Model file for the job. Use its own axes, mm. A direction names the side the tool comes from. Give positions to 0.01 mm unless a question says otherwise; leave off trailing zeros. Loops run counter-clockwise (first coordinate to the right, second up) from the corner with the lowest first, then second, coordinate; pieces in that order, holes last. Notation, with made-up numbers: (13.25, 63.25) -> (42.25, 63.25) arc R30 ccw to (42.25, 96.25) -> close; hole circle Ø9 at (-7.5, 18.25). An arc over 180 degrees is marked (long way). Use CSV: the item, a comma, the result in double quotes. Start each with the question number.
(1) Drill centre lines: probe 1 along Z at (x, y) = (-5.5, 0.25); probe 2 along Y at (x, z) = (0, 8); probe 3 along X at (y, z) = (2, 7.25). Where is each one in solid material? Low to high.
(2) 3-axis set-ups, long thin cutter, end or side, ignore diameter. For faces 1 (the cylindrical face through (-0.45, 4.62, 1.82)), 2 (the cylindrical face through (-2.38, 3.82, 10.44)), 3 (the cylindrical face through (-6.466, 2.681, 3.204)), 4 (the cylindrical face through (0, -4.5, 10.4)): which of +Z, -Z, +X, -X, +Y, -Y reach the whole face in a straight line?
(3) Cut at A-A on x = 0. Write the cut outline in (y, z), then the cut area to 3 significant figures.
(4) Cut at C-C on y = -2.25. Write the cut outline in (x, z).
(5) Pull direction Z, two halves, no side cores. Call faces 5 (the flat face through (-3, 0, 16)), 6 (the cylindrical face through (-6.466, 2.681, 15.24)), 7 (the cylindrical face through (-0.841, 4.422, 10.444)): pulls with the +Z half, pulls with the -Z half, needs draft (parallel to the pull), parting line crosses it, or undercut.
(6) Flat gauge pins, fed straight in: pin 1 (7 mm diameter, centred on x = -1, y = 0, fed in from +Z); pin 2 (2 mm diameter, centred on x = -3, z = 14, fed in from +Y); pin 3 (6 mm diameter, centred on x = 3.5, z = 5.5, fed in from +Y); pin 4 (1.8 mm diameter, centred on x = 0, z = 3.25, fed in from +Y). Where does each tip first touch, or does it go through?
(7) Cut at B-B on y = 5.5. Write the cut outline in (x, z), then the cut area to 3 significant figures.
(8) Cut at D-D on x = -5.75. Write the cut outline in (y, z), then the cut area to 3 significant figures.
from build123d import *

# Parameters (mm, degrees)
ESQUISSE1_R                  = 7
BOSS_EXTRU_1_DEPTH           = 6.5
BOSS_EXTRU_2_DEPTH           = 8
ESQUISSE4_R                  = 7
BOSS_EXTRU_3_DEPTH           = 1.5
ESQUISSE5_R                  = 2.75
ENL_V_MAT_EXTRU_1_DEPTH      = 16
ENL_V_MAT_EXTRU_3_REACH      = 20.815
ENL_V_MAT_EXTRU_3_END_RADIUS = 7
ESQUISSE8_R                  = 1.5


with BuildPart() as part:
    # Esquisse1 → Boss.-Extru.1 (new body)
    with BuildSketch(Plane.XY):
        with Locations(Location((0, 0, 0), (0, 0, 180))):
            Circle(ESQUISSE1_R)
    extrude(amount=BOSS_EXTRU_1_DEPTH)

    # Esquisse3 → Boss.-Extru.2 (add)
    with BuildSketch(Plane.XY.offset(6.5)):
        with BuildLine():
            Line((0, 5.194220739), (0.3, 5.194220739))
            ThreePointArc((0.3, 5.194220739), (0.827122819, 4.424716273), (1.596627286, 4.951839093))
            Line((1.596627286, 4.951839093), (1.876368954, 4.843466593))
            Line((1.876368954, 4.843466593), (2.156110623, 4.735094093))
            ThreePointArc((2.156110623, 4.735094093), (2.369660938, 3.827133822), (3.277621209, 4.040684138))
            Line((3.277621209, 4.040684138), (3.499323884, 3.838575444))
            Line((3.499323884, 3.838575444), (3.721026559, 3.636466751))
            ThreePointArc((3.721026559, 3.636466751), (3.592163217, 2.712675742), (4.515954226, 2.583812399))
            Line((4.515954226, 2.583812399), (4.649675733, 2.315263412))
            Line((4.649675733, 2.315263412), (4.78339724, 2.046714425))
            ThreePointArc((4.78339724, 2.046714425), (4.329523948, 1.231855771), (5.144382602, 0.777982479))
            Line((5.144382602, 0.777982479), (5.172063109, 0.479262226))
            Line((5.172063109, 0.479262226), (5.199743617, 0.180541973))
            ThreePointArc((5.199743617, 0.180541973), (4.482158479, -0.415333148), (5.0780336, -1.132918286))
            Line((5.0780336, -1.132918286), (4.995934703, -1.421465979))
            Line((4.995934703, -1.421465979), (4.913835806, -1.710013672))
            ThreePointArc((4.913835806, -1.710013672), (4.029452671, -2.006429023), (4.325868023, -2.890812158))
            Line((4.325868023, -2.890812158), (4.145077632, -3.130217327))
            Line((4.145077632, -3.130217327), (3.964287241, -3.369622495))
            ThreePointArc((3.964287241, -3.369622495), (3.032546952, -3.326545541), (2.989469999, -4.258285831))
            Line((2.989469999, -4.258285831), (2.734404858, -4.416215479))
            Line((2.734404858, -4.416215479), (2.479339718, -4.574145128))
            ThreePointArc((2.479339718, -4.574145128), (1.626078963, -4.197393651), (1.249327486, -5.050654405))
            Line((1.249327486, -5.050654405), (0.954435556, -5.105779261))
            Line((0.954435556, -5.105779261), (0.659543626, -5.160904116))
            ThreePointArc((0.659543626, -5.160904116), (0, -4.50136049), (-0.659543626, -5.160904116))
            Line((-0.659543626, -5.160904116), (-0.954435556, -5.105779261))
            Line((-0.954435556, -5.105779261), (-1.249327486, -5.050654405))
            ThreePointArc((-1.249327486, -5.050654405), (-1.626078963, -4.197393651), (-2.479339718, -4.574145128))
            Line((-2.479339718, -4.574145128), (-2.734404858, -4.416215479))
            Line((-2.734404858, -4.416215479), (-2.989469999, -4.258285831))
            ThreePointArc((-2.989469999, -4.258285831), (-3.032546952, -3.326545541), (-3.964287241, -3.369622495))
            Line((-3.964287241, -3.369622495), (-4.145077632, -3.130217327))
            Line((-4.145077632, -3.130217327), (-4.325868023, -2.890812158))
            ThreePointArc((-4.325868023, -2.890812158), (-4.029452671, -2.006429023), (-4.913835806, -1.710013672))
            Line((-4.913835806, -1.710013672), (-4.995934703, -1.421465979))
            Line((-4.995934703, -1.421465979), (-5.0780336, -1.132918286))
            ThreePointArc((-5.0780336, -1.132918286), (-4.482158479, -0.415333148), (-5.199743617, 0.180541973))
            Line((-5.199743617, 0.180541973), (-5.172063109, 0.479262226))
            Line((-5.172063109, 0.479262226), (-5.144382602, 0.777982479))
            ThreePointArc((-5.144382602, 0.777982479), (-4.329523948, 1.231855771), (-4.78339724, 2.046714425))
            Line((-4.78339724, 2.046714425), (-4.649675733, 2.315263412))
            Line((-4.649675733, 2.315263412), (-4.515954226, 2.583812399))
            ThreePointArc((-4.515954226, 2.583812399), (-3.592163217, 2.712675742), (-3.721026559, 3.636466751))
            Line((-3.721026559, 3.636466751), (-3.499323884, 3.838575444))
            Line((-3.499323884, 3.838575444), (-3.277621209, 4.040684138))
            ThreePointArc((-3.277621209, 4.040684138), (-2.369660938, 3.827133822), (-2.156110623, 4.735094093))
            Line((-2.156110623, 4.735094093), (-1.876368954, 4.843466593))
            Line((-1.876368954, 4.843466593), (-1.596627286, 4.951839093))
            ThreePointArc((-1.596627286, 4.951839093), (-0.827122819, 4.424716273), (-0.3, 5.194220739))
            Line((-0.3, 5.194220739), (0, 5.194220739))
        make_face()
    extrude(amount=BOSS_EXTRU_2_DEPTH)

    # Esquisse4 → Boss.-Extru.3 (add)
    with BuildSketch(Plane.XY.offset(14.5)):
        with Locations(Location((0, 0, 0), (0, 0, 180))):
            Circle(ESQUISSE4_R)
    extrude(amount=BOSS_EXTRU_3_DEPTH)

    # Esquisse5 → Enlèv. mat.-Extru.1 (cut)
    with BuildSketch(Plane(origin=(0, 0, 0), x_dir=(-1, 0, 0), z_dir=(0, 0, -1))):
        Circle(ESQUISSE5_R)
    extrude(amount=-ENL_V_MAT_EXTRU_1_DEPTH, mode=Mode.SUBTRACT)

    # Enlèv. mat.-Extru.3: up to this cylinder (the profile starts inside it)
    enl_v_mat_extru_3_end = Plane(origin=(0, 0, 3.25), z_dir=(0, 0, -1)) * Cylinder(ENL_V_MAT_EXTRU_3_END_RADIUS, 56.63, mode=Mode.PRIVATE)
    # Esquisse8 → Enlèv. mat.-Extru.3 (cut, up to the surface)
    with BuildSketch(Plane(origin=(0, 0, 0), x_dir=(1, 0, 0), z_dir=(0, 1, 0)), mode=Mode.PRIVATE) as enl_v_mat_extru_3_sk1:
        with Locations(Location((0, -3.25, 0), (0, 0, 90))):
            Circle(ESQUISSE8_R)
    enl_v_mat_extru_3_tool1 = extrude(enl_v_mat_extru_3_sk1.sketch, amount=ENL_V_MAT_EXTRU_3_REACH, mode=Mode.PRIVATE) & enl_v_mat_extru_3_end
    add(enl_v_mat_extru_3_tool1.solids().sort_by_distance((0, 0, 3.25))[0], mode=Mode.SUBTRACT)


solid = part.part
Check result:
1,probe 1,"0 to 6.5, 14.5 to 16"
1,probe 2,"-4.5 to -2.75, 2.75 to 5.19"
1,probe 3,"-4.66 to -1.89, 1.89 to 4.66"
2,face 1,"+Y"
2,face 2,"none"
2,face 3,"+Z, -Z"
2,face 4,"-Y"
3,outline,"(-7, 0) -> (-2.75, 0) -> (-2.75, 16) -> (-7, 16) -> (-7, 14.5) -> (-4.5, 14.5) -> (-4.5, 6.5) -> (-7, 6.5) -> close; (2.75, 0) -> (7, 0) -> (7, 1.75) -> (2.75, 1.75) -> close; (2.75, 4.75) -> (7, 4.75) -> (7, 6.5) -> (5.19, 6.5) -> (5.19, 14.5) -> (7, 14.5) -> (7, 16) -> (2.75, 16) -> close"
3,area,"88.8 mm²"
4,outline,"(-6.63, 0) -> (-1.58, 0) -> (-1.58, 16) -> (-6.63, 16) -> (-6.63, 14.5) -> (-3.96, 14.5) -> (-3.96, 6.5) -> (-6.63, 6.5) -> close; (1.58, 0) -> (6.63, 0) -> (6.63, 6.5) -> (3.96, 6.5) -> (3.96, 14.5) -> (6.63, 14.5) -> (6.63, 16) -> (1.58, 16) -> close"
5,face 5,"pulls with the +Z half"
5,face 6,"needs draft"
5,face 7,"undercut"
6,pin 1,"z = 16"
6,pin 2,"y = 6.67"
6,pin 3,"y = 6.98"
6,pin 4,"y = -2.6"
7,outline,"(-4.33, 0) -> (4.33, 0) -> (4.33, 6.5) -> (-4.33, 6.5) -> close; (-4.33, 14.5) -> (4.33, 14.5) -> (4.33, 16) -> (-4.33, 16) -> close; hole circle Ø3 at (0, 3.25)"
7,area,"62.2 mm²"
8,outline,"(-3.99, 0) -> (3.99, 0) -> (3.99, 6.5) -> (-3.99, 6.5) -> close; (-3.99, 14.5) -> (3.99, 14.5) -> (3.99, 16) -> (-3.99, 16) -> close"
8,area,"63.9 mm²"
